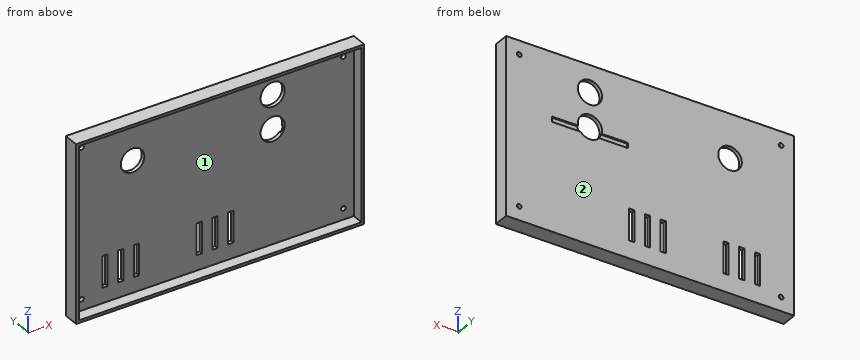
```python
from build123d import *

# Parameters (mm, degrees)
SKETCH_1_W                       = 220
SKETCH_1_H                       = 135
LID_TOP_3MM_DEPTH                = 3
SKETCH_2_W                       = 216
SKETCH_2_H                       = 2
LID_RIM_BACK_DEPTH               = 12
SKETCH_3_W                       = 216
SKETCH_3_H                       = 2
LID_RIM_FRONT_DEPTH              = 12
SKETCH_4_W                       = 2
SKETCH_4_H                       = 135
LID_RIM_LEFT_DEPTH               = 12
SKETCH_5_W                       = 2
SKETCH_5_H                       = 135
LID_RIM_RIGHT_DEPTH              = 12
SKETCH_6_R                       = 1.8
LID_SCREW_CLEARANCE_1_DEPTH      = 16
SKETCH_7_R                       = 1.8
LID_SCREW_CLEARANCE_2_DEPTH      = 16
SKETCH_8_R                       = 1.8
LID_SCREW_CLEARANCE_3_DEPTH      = 16
SKETCH_9_R                       = 1.8
LID_SCREW_CLEARANCE_4_DEPTH      = 16
SKETCH_10_R                      = 9
OV5647_LENS_OPENING_D18_DEPTH    = 4
SKETCH_11_R                      = 9.25
HC_SR04_ACOUSTIC_OPENING_1_DEPTH = 4
SKETCH_12_R                      = 9.25
HC_SR04_ACOUSTIC_OPENING_2_DEPTH = 4
SKETCH_13_W                      = 58
SKETCH_13_H                      = 4
HC_SR04_ALIGNMENT_RECESS_DEPTH   = 1.2
SKETCH_14_W                      = 4
SKETCH_14_H                      = 24
VENT_SLOT_1_DEPTH                = 4
SKETCH_15_W                      = 4
SKETCH_15_H                      = 24
VENT_SLOT_2_DEPTH                = 4
SKETCH_16_W                      = 4
SKETCH_16_H                      = 24
VENT_SLOT_3_DEPTH                = 4
SKETCH_17_W                      = 4
SKETCH_17_H                      = 24
VENT_SLOT_4_DEPTH                = 4
SKETCH_18_W                      = 4
SKETCH_18_H                      = 24
VENT_SLOT_5_DEPTH                = 4
SKETCH_19_W                      = 4
SKETCH_19_H                      = 24
VENT_SLOT_6_DEPTH                = 4


with BuildPart() as part:
    # 草图1 → Lid_Top_3mm (new body)
    with BuildSketch(Plane(origin=(0, 0, 0), x_dir=(1, 0, 0), z_dir=(0, 1, 0))):
        Rectangle(SKETCH_1_W, SKETCH_1_H)
    extrude(amount=-LID_TOP_3MM_DEPTH)

    # 草图2 → Lid_Rim_Back (add)
    with BuildSketch(Plane(origin=(0, 0, 0), x_dir=(1, 0, 0), z_dir=(0, 1, 0))):
        with Locations((0, 66.5)):
            Rectangle(SKETCH_2_W, SKETCH_2_H)
    extrude(amount=-LID_RIM_BACK_DEPTH)

    # 草图3 → Lid_Rim_Front (add)
    with BuildSketch(Plane(origin=(0, 0, 0), x_dir=(1, 0, 0), z_dir=(0, 1, 0))):
        with Locations((0, -66.5)):
            Rectangle(SKETCH_3_W, SKETCH_3_H)
    extrude(amount=-LID_RIM_FRONT_DEPTH)

    # 草图4 → Lid_Rim_Left (add)
    with BuildSketch(Plane(origin=(0, 0, 0), x_dir=(1, 0, 0), z_dir=(0, 1, 0))):
        with Locations((-109, 0)):
            Rectangle(SKETCH_4_W, SKETCH_4_H)
    extrude(amount=-LID_RIM_LEFT_DEPTH)

    # 草图5 → Lid_Rim_Right (add)
    with BuildSketch(Plane(origin=(0, 0, 0), x_dir=(1, 0, 0), z_dir=(0, 1, 0))):
        with Locations((109, 0)):
            Rectangle(SKETCH_5_W, SKETCH_5_H)
    extrude(amount=-LID_RIM_RIGHT_DEPTH)

    # 草图6 → Lid_Screw_Clearance_1 (cut)
    with BuildSketch(Plane(origin=(0, 0, 0), x_dir=(1, 0, 0), z_dir=(0, 1, 0))):
        with Locations(Location((-100, -57, 0), (0, 0, 270))):
            Circle(SKETCH_6_R)
    extrude(amount=-LID_SCREW_CLEARANCE_1_DEPTH, mode=Mode.SUBTRACT)

    # 草图7 → Lid_Screw_Clearance_2 (cut)
    with BuildSketch(Plane(origin=(0, 0, 0), x_dir=(1, 0, 0), z_dir=(0, 1, 0))):
        with Locations(Location((100, -57, 0), (0, 0, 270))):
            Circle(SKETCH_7_R)
    extrude(amount=-LID_SCREW_CLEARANCE_2_DEPTH, mode=Mode.SUBTRACT)

    # 草图8 → Lid_Screw_Clearance_3 (cut)
    with BuildSketch(Plane(origin=(0, 0, 0), x_dir=(1, 0, 0), z_dir=(0, 1, 0))):
        with Locations(Location((-100, 57, 0), (0, 0, 270))):
            Circle(SKETCH_8_R)
    extrude(amount=-LID_SCREW_CLEARANCE_3_DEPTH, mode=Mode.SUBTRACT)

    # 草图9 → Lid_Screw_Clearance_4 (cut)
    with BuildSketch(Plane(origin=(0, 0, 0), x_dir=(1, 0, 0), z_dir=(0, 1, 0))):
        with Locations(Location((100, 57, 0), (0, 0, 270))):
            Circle(SKETCH_9_R)
    extrude(amount=-LID_SCREW_CLEARANCE_4_DEPTH, mode=Mode.SUBTRACT)

    # 草图10 → OV5647_Lens_Opening_D18 (cut)
    with BuildSketch(Plane(origin=(0, 0, 0), x_dir=(1, 0, 0), z_dir=(0, 1, 0))):
        with Locations(Location((-61, -34, 0), (0, 0, 270))):
            Circle(SKETCH_10_R)
    extrude(amount=-OV5647_LENS_OPENING_D18_DEPTH, mode=Mode.SUBTRACT)

    # 草图11 → HC_SR04_Acoustic_Opening_1 (cut)
    with BuildSketch(Plane(origin=(0, 0, 0), x_dir=(1, 0, 0), z_dir=(0, 1, 0))):
        with Locations(Location((46, -47, 0), (0, 0, 270))):
            Circle(SKETCH_11_R)
    extrude(amount=-HC_SR04_ACOUSTIC_OPENING_1_DEPTH, mode=Mode.SUBTRACT)

    # 草图12 → HC_SR04_Acoustic_Opening_2 (cut)
    with BuildSketch(Plane(origin=(0, 0, 0), x_dir=(1, 0, 0), z_dir=(0, 1, 0))):
        with Locations(Location((46, -21, 0), (0, 0, 270))):
            Circle(SKETCH_12_R)
    extrude(amount=-HC_SR04_ACOUSTIC_OPENING_2_DEPTH, mode=Mode.SUBTRACT)

    # 草图13 → HC_SR04_Alignment_Recess (cut)
    with BuildSketch(Plane(origin=(0, 0, 0), x_dir=(1, 0, 0), z_dir=(0, 1, 0))):
        with Locations((46, -17)):
            Rectangle(SKETCH_13_W, SKETCH_13_H)
    extrude(amount=-HC_SR04_ALIGNMENT_RECESS_DEPTH, mode=Mode.SUBTRACT)

    # 草图14 → Vent_Slot_1 (cut)
    with BuildSketch(Plane(origin=(0, 0, 0), x_dir=(1, 0, 0), z_dir=(0, 1, 0))):
        with Locations((-82, 42)):
            Rectangle(SKETCH_14_W, SKETCH_14_H)
    extrude(amount=-VENT_SLOT_1_DEPTH, mode=Mode.SUBTRACT)

    # 草图15 → Vent_Slot_2 (cut)
    with BuildSketch(Plane(origin=(0, 0, 0), x_dir=(1, 0, 0), z_dir=(0, 1, 0))):
        with Locations((-70, 42)):
            Rectangle(SKETCH_15_W, SKETCH_15_H)
    extrude(amount=-VENT_SLOT_2_DEPTH, mode=Mode.SUBTRACT)

    # 草图16 → Vent_Slot_3 (cut)
    with BuildSketch(Plane(origin=(0, 0, 0), x_dir=(1, 0, 0), z_dir=(0, 1, 0))):
        with Locations((-58, 42)):
            Rectangle(SKETCH_16_W, SKETCH_16_H)
    extrude(amount=-VENT_SLOT_3_DEPTH, mode=Mode.SUBTRACT)

    # 草图17 → Vent_Slot_4 (cut)
    with BuildSketch(Plane(origin=(0, 0, 0), x_dir=(1, 0, 0), z_dir=(0, 1, 0))):
        with Locations((-10, 42)):
            Rectangle(SKETCH_17_W, SKETCH_17_H)
    extrude(amount=-VENT_SLOT_4_DEPTH, mode=Mode.SUBTRACT)

    # 草图18 → Vent_Slot_5 (cut)
    with BuildSketch(Plane(origin=(0, 0, 0), x_dir=(1, 0, 0), z_dir=(0, 1, 0))):
        with Locations((2, 42)):
            Rectangle(SKETCH_18_W, SKETCH_18_H)
    extrude(amount=-VENT_SLOT_5_DEPTH, mode=Mode.SUBTRACT)

    # 草图19 → Vent_Slot_6 (cut)
    with BuildSketch(Plane(origin=(0, 0, 0), x_dir=(1, 0, 0), z_dir=(0, 1, 0))):
        with Locations((14, 42)):
            Rectangle(SKETCH_19_W, SKETCH_19_H)
    extrude(amount=-VENT_SLOT_6_DEPTH, mode=Mode.SUBTRACT)


solid = part.part
```
Could you check a few things on this model? Use its own coordinates, in mm. Face numbers are marked on the shaded views. Coordinates: 2 decimals unless noted, no trailing zeros. Write each loop counter-clockwise with the first axis right and the second up, starting at its lowest first coordinate (ties: lowest second). Pieces come first, ordered by that corner, then holes. Notation, with made-up numbers: (72.5, 17) -> (81.5, 17) arc R13 cw to (81.5, 38) -> close; hole circle Ø5 at (-24.75, 73.5). An arc over 180 degrees is marked (long way). Return JSON: item names as keys, results as strings.
(1) Imagine slicing it at B-B, the plane x = 46. Please give me the cut outline in (y, z), then the cut area to 3 significant figures.
Numbers:
{"outline": "(-12, -67.5) -> (0, -67.5) -> (0, 11.75) -> (-3, 11.75) -> (-3, -65.5) -> (-12, -65.5) -> close; (-12, 65.5) -> (-3, 65.5) -> (-3, 56.25) -> (0, 56.25) -> (0, 67.5) -> (-12, 67.5) -> close; (-3, 30.25) -> (0, 30.25) -> (0, 37.75) -> (-3, 37.75) -> close", "area": "330 mm2"}
(2) I need wall thicknesses on L1, parallel to X at y = -1.75, z = -57; L2, parallel to Z at x = 78, y = -11; L3, parallel to X at y = -2.3, z = 34. Which ranges of each line are inside material? Lowest first, please.
Numbers:
{"L1": "x = -110 to -101.8, -98.2 to 98.2, 101.8 to 110", "L2": "z = -67.5 to -65.5, 65.5 to 67.5", "L3": "x = -110 to -70, -52 to 110"}
(3) I'm going to push flat-ended pins straight in: pin 1 (5 mm diameter, centred on x = 78, z = -47, fed in from -Y); pin 2 (2 mm diameter, centred on x = 65.5, z = 16.5, fed in from +Y). Where does each tip first touch, or does it pass through?
Numbers:
{"pin 1": "stops at y = -3", "pin 2": "stops at y = -1.2"}
(4) Imagine slicing it at C-C, the plane z = 47. Please give me the cut outline in (x, y).
Numbers:
{"outline": "(-110, -12) -> (-108, -12) -> (-108, -3) -> (36.75, -3) -> (36.75, 0) -> (-110, 0) -> close; (55.25, -3) -> (108, -3) -> (108, -12) -> (110, -12) -> (110, 0) -> (55.25, 0) -> close"}
(5) Imagine slicing it at A-A, the plane z = -37.5. Count the separate pieces of the cut face and the enclosed holes in it, then the cut area to 3 significant figures.
Numbers:
{"separate pieces": "7", "enclosed holes": "0", "area": "624 mm2"}
(6) We'd pull the mould along Z, two halves only. Please class the marked faces 1 and 2: +Z half, -Z half, draft (parallel to the pull), parting line (faces both ways), or undercut.
Numbers:
{"face 1": "undercut", "face 2": "draft"}
(7) Imagine slicing it at D-D, the plane y = -7.5. Please give me the cut outline in (x, z).
Numbers:
{"outline": "(-110, -67.5) -> (110, -67.5) -> (110, 67.5) -> (-110, 67.5) -> close; hole (-108, -65.5) -> (108, -65.5) -> (108, 65.5) -> (-108, 65.5) -> close"}
